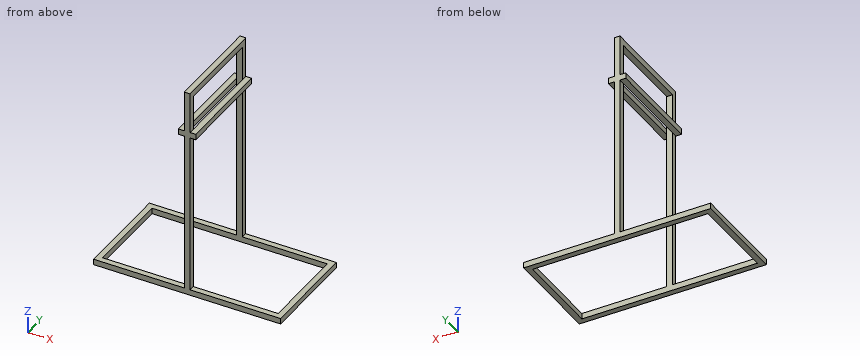
```python
from build123d import *

# Parameters (mm, degrees)
F0_W      = 25.4
F0_H      = 25.4
F1_DEPTH  = 25.4
F0_H_2    = 387.35
F2_DEPTH  = 939.8
F4_DEPTH  = 25.4
F7_W      = 25.4
F7_H      = 25.4
F7_W_2    = 387.35
F8_DEPTH  = 25.4
F9_W      = 438.15
F9_H      = 25.4
F10_DEPTH = 25.4


# Not quite as in the source:
# - the program builds the solid bodies; features that only make, move or delete a surface that nothing else refers to are left out


with BuildPart() as f1:
    # F0 (on Top) → F1 (new body)
    with BuildSketch(Plane.XY):
        Polygon((412.75, -219.075), (412.75, 219.075), (38.1, 219.075), (38.1, 193.675), (387.35, 193.675), (387.35, -193.675), (38.1, -193.675), (38.1, -219.075), align=None)
        with Locations((25.4, 206.375)):
            Rectangle(F0_W, F0_H)
        with Locations((0, 206.375)):
            Rectangle(F0_W, F0_H)
        with Locations((25.4, -206.375)):
            Rectangle(F0_W, F0_H)
        with Locations((-25.4, 206.375)):
            Rectangle(F0_W, F0_H)
        with Locations((0, -206.375)):
            Rectangle(F0_W, F0_H)
        Polygon((-38.1, 193.675), (-38.1, 219.075), (-412.75, 219.075), (-412.75, -219.075), (-38.1, -219.075), (-38.1, -193.675), (-387.35, -193.675), (-387.35, 193.675), align=None)
        with Locations((-25.4, -206.375)):
            Rectangle(F0_W, F0_H)
    extrude(amount=F1_DEPTH)

    # F0 (on Top) → F2 (join)
    with BuildSketch(Plane.XY):
        Rectangle(F0_W, F0_H_2)
        with Locations((0, 206.375)):
            Rectangle(F0_W, F0_H)
        with Locations((0, -206.375)):
            Rectangle(F0_W, F0_H)
    extrude(amount=F2_DEPTH)

    # F3 (on face) → F4 (cut)
    with BuildSketch(Plane(origin=(-12.7, 0, 0), x_dir=(0, -1, 0), z_dir=(-1, 0, 0))):
        Polygon((-193.675, -2.54), (193.675, -2.54), (193.675, 737.5616856575), (193.675, 911.86), (-193.675, 911.86), (-193.675, 737.5616856575), align=None)
    extrude(amount=-F4_DEPTH, mode=Mode.SUBTRACT)

    # F7 (on face) → F8 (join)
    with BuildSketch(Plane(origin=(-12.7, 0, 0), x_dir=(0, -1, 0), z_dir=(-1, 0, 0))):
        with Locations((206.375, 746.76)):
            Rectangle(F7_W, F7_H)
        with Locations((0, 746.76)):
            Rectangle(F7_W_2, F7_H)
        with Locations((-206.375, 746.76)):
            Rectangle(F7_W, F7_H)
    extrude(amount=F8_DEPTH)

    # F9 (on face) → F10 (join)
    with BuildSketch(Plane.YZ.offset(12.7)):
        with Locations((0, 746.9166304588)):
            Rectangle(F9_W, F9_H)
    extrude(amount=F10_DEPTH)


solid = f1.part
```
Geometry check sheet. Reference: the model listing, model coordinates, mm. Coordinates: 2 decimals unless noted, no trailing zeros. Order: outer loops, then holes, each group sorted by start corner. A loop starts at its lowest first (then second) coordinate and runs counter-clockwise, first axis right, second up. Notation, with made-up numbers: (71.25, 13.25) - (107.25, 13.25) arc R9 cw to (107.25, 23.25) - close; hole circle Ø6 at (-1.5, 37). An arc over 180 degrees is marked (long way). Use one line per item in the form item = value.
1. Gauge pin test, flat ends, axial feed: pin 1 (7.5 mm diameter, centred on x = -28, y = 21, fed in from +Z); pin 2 (12.5 mm diameter, centred on x = 22.5, y = -69, fed in from +Z); pin 3 (12.5 mm diameter, centred on y = 208, z = 267, fed in from +X). Record the tip position at first contact, or that the pin passes through.
Here are the results:
pin_1 = 759.46
pin_2 = 759.62
pin_3 = 12.7
2. Section check A-A (z = 465). Record the boundary of the cut face in (x, y) (3 decimals).
Here are the results:
outline = (-12.7, -219.075) - (12.7, -219.075) - (12.7, -193.675) - (-12.7, -193.675) - close; (-12.7, 193.675) - (12.7, 193.675) - (12.7, 219.075) - (-12.7, 219.075) - close
3. Section check B-B (x = 346.5). Record the boundary of the cut face in (y, z) (3 decimals), then the cut area to 3 significant figures.
Here are the results:
outline = (-219.075, 0) - (-193.675, 0) - (-193.675, 25.4) - (-219.075, 25.4) - close; (193.675, 0) - (219.075, 0) - (219.075, 25.4) - (193.675, 25.4) - close
area = 1,290 mm²
4. Section check C-C (y = -165). Record the boundary of the cut face in (x, z).
Here are the results:
outline = (-412.75, 0) - (-387.35, 0) - (-387.35, 25.4) - (-412.75, 25.4) - close; (-38.1, 734.06) - (-12.7, 734.06) - (-12.7, 759.46) - (-38.1, 759.46) - close; (-12.7, 911.86) - (12.7, 911.86) - (12.7, 939.8) - (-12.7, 939.8) - close; (12.7, 734.22) - (38.1, 734.22) - (38.1, 759.62) - (12.7, 759.62) - close; (387.35, 0) - (412.75, 0) - (412.75, 25.4) - (387.35, 25.4) - close
5. Scan line: line 1 (X direction, y = 146, z = 746). Record every from-to range of solid material in increasing order.
Here are the results:
line_1 = -38.1 to -12.7, 12.7 to 38.1
